Can you work these out from the model? Positions are in its coordinate system, mm. A direction names the side the tool comes from. Round coordinates to 2 decimals unless told otherwise and drop trailing zeros. Order: outer loops, then holes, each group sorted by start corner. A loop starts at its lowest first (then second) coordinate and runs counter-clockwise, first axis right, second up.
Q1. If we section it at C-C (x = 4): Please give me the cut outline in (y, z).
Q2. If I drill on line 1 (X direction, y = -185, z = 31); line 2 (Y direction, x = 0, z = 35.5); line 3 (Y direction, x = 8, z = 26), over which ranges is the centre line in solid material (lowest first)?
Q3. If we section it at D-D (y = -47): Please give me the cut outline in (x, z), plus the area to 3 significant figures.
Q4. Will these pins go through, and if not, where does the flat tip stop? P1, Ø5.5, axis at x = -19, z = 20, coming from the -Y side; P2, Ø12, axis at x = -3, y = -113, coming from the -Z side; P3, Ø3.5, axis at x = 8, y = 0, coming from the -Z side; P4, Ø3.5, axis at x = -17, z = 12, coming from the +Y side.
Q5. For faces 4 (the face through (-19, -85, 15)), 5 (the face through (-14, -103, 15)), 6 (the face through (-1, -5, 15)), which set-ups out of +Z, -Z, +X, -X, +Y, -Y let a thin tool reach every point of the face, with its end or its side?
Q6. If we section it at B-B (z = 34.5): Please give me the cut outline in (x, y), plus the area to 3 significant figures.
Q7. If we section it at A-A (z = 7): Count the separate pieces of the cut face and the enclosed holes in it, plus the area to 3 significant figures.
Q8. We'd pull the mould along Y, two halves only. Please class faces 1 (the face through (8.15, -196.99, 25.35)), 2 (the face through (-7, -187, 0)), 3 (the face through (-7, -175, 15)): pulls with the +Y half, pulls with the -Y half, needs draft (parallel to the pull), parting line crosses it, or undercut.
from build123d import *

# Parameters (mm, degrees)
CROQUIS1_R              = 1.5
SALIENTE_EXTRUIR1_DEPTH = 50
CORTAR_EXTRUIR1_REACH   = 211.275
CROQUIS2_W              = 30
CROQUIS2_H              = 170
REDONDEO1_R             = 10
REDONDEO2_R             = 10
CROQUIS3_W              = 11
CROQUIS3_H              = 35
CROQUIS3_R              = 1.5
SALIENTE_EXTRUIR2_DEPTH = 30


with BuildPart() as part:
    # Croquis1 → Saliente-Extruir1 (new body)
    with BuildSketch(Plane(origin=(0, 0, 0), x_dir=(0, 1, 0), z_dir=(0, 0, 1))):
        Polygon((-85, 25), (10, 10), (10, -11), (-200, -11), (-200, 25), align=None)
        with Locations(Location((0, 0, 0), (0, 0, 270))):
            Circle(CROQUIS1_R, mode=Mode.SUBTRACT)
        with Locations(Location((-185, 0, 0), (0, 0, 270))):
            Circle(CROQUIS1_R, mode=Mode.SUBTRACT)
        with Locations(Location((-185, 15, 0), (0, 0, 270))):
            Circle(CROQUIS1_R, mode=Mode.SUBTRACT)
        with Locations(Location((0, -8, 0), (0, 0, 270))):
            Circle(CROQUIS1_R, mode=Mode.SUBTRACT)
    extrude(amount=SALIENTE_EXTRUIR1_DEPTH)

    # Croquis2 → Cortar-Extruir1 (cut, up to next)
    with BuildSketch(Plane(origin=(11, 0, 0), x_dir=(0, 0, -1), z_dir=(1, 0, 0)), mode=Mode.PRIVATE) as cortar_extruir1_sk1:
        with Locations((-15, -90)):
            Rectangle(CROQUIS2_W, CROQUIS2_H)
    cortar_extruir1_tool1 = extrude(cortar_extruir1_sk1.sketch, amount=-CORTAR_EXTRUIR1_REACH, mode=Mode.PRIVATE) & part.part
    add(cortar_extruir1_tool1.solids().sort_by_distance((11, -90, 15))[0], mode=Mode.SUBTRACT)

    # Redondeo1
    redondeo1_edges = [part.edges().sort_by_distance(p)[0] for p in [
        (11, -200, 25),
        (-25, -200, 25),
    ]]
    fillet(redondeo1_edges, radius=REDONDEO1_R)

    # Redondeo2
    redondeo2_edges = [part.edges().sort_by_distance(p)[0] for p in [
        (-10, 10, 25),
    ]]
    fillet(redondeo2_edges, radius=REDONDEO2_R)

    # Croquis3 → Saliente-Extruir2 (add)
    with BuildSketch(Plane(origin=(0, 0, 30), x_dir=(-1, 0, 0), z_dir=(0, 0, -1))):
        with Locations((19.5, -102.5)):
            Rectangle(CROQUIS3_W, CROQUIS3_H)
        with Locations(Location((19, -90, 0), (0, 0, 90))):
            Circle(CROQUIS3_R, mode=Mode.SUBTRACT)
        with Locations(Location((19, -110, 0), (0, 0, 90))):
            Circle(CROQUIS3_R, mode=Mode.SUBTRACT)
    extrude(amount=SALIENTE_EXTRUIR2_DEPTH)


solid = part.part
Solution:
1. outline: (-199.54, 0) - (-175, 0) - (-175, 30) - (-5, 30) - (-5, 0) - (10, 0) - (10, 50) - (-199.54, 50) - close
2. line 1: x = -25 to -16.5, -13.5 to -1.5, 1.5 to 11
2. line 2: y = -200 to -186.5, -183.5 to -1.5, 1.5 to 10
2. line 3: y = -197.14 to -175, -5 to -1.5, 1.5 to 10
3. outline: (-19, 30) - (11, 30) - (11, 50) - (-19, 50) - close
3. area: 600 mm2
4. P1: stops at y = -199.92
4. P2: stops at z = 30
4. P3: stops at z = 0
4. P4: stops at y = -85
5. face 4: -Z, +X, -X, +Y
5. face 5: -Z, +X, +Y
5. face 6: -Z, +X, -X
6. outline: (-25, -190) arc R10 ccw to (-15, -200) - (1, -200) arc R10 ccw to (11, -190) - (11, 10) - (-1.46, 10) arc R10 ccw to (-11.33, 1.56) - (-25, -85) - close; hole circle Ø3 at (-15, -185); hole circle Ø3 at (0, -185); hole circle Ø3 at (0, 0); hole circle Ø3 at (8, 0)
6. area: 6,760 mm2
7. separate pieces: 3
7. enclosed holes: 6
7. area: 1,520 mm2
8. face 1: pulls with the -Y half
8. face 2: needs draft
8. face 3: undercut
